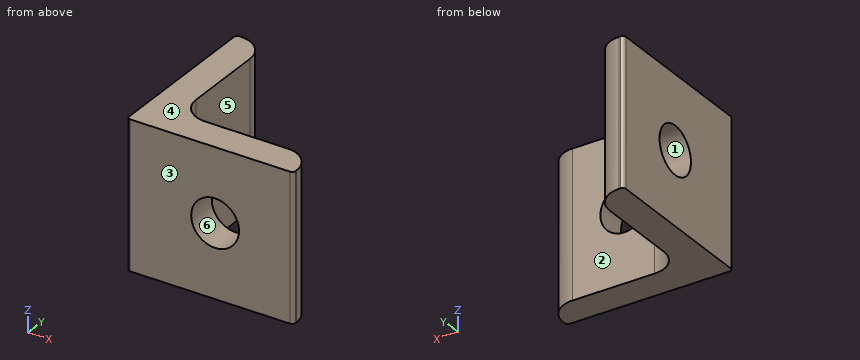
```python
from build123d import *

# Parameters (mm, degrees)
BOSS_EXTRUDE1_DEPTH = 22
SKETCH2_R           = 3.59
CUT_EXTRUDE1_DEPTH  = 42.641325627
SKETCH3_R           = 3.59
CUT_EXTRUDE2_DEPTH  = 42.641325627
FILLET1_R           = 4
FILLET2_R           = 0.5


with BuildPart() as part:
    # Sketch1 → Boss-Extrude1 (new body)
    with BuildSketch(Plane.XY):
        Polygon((0, 0), (25, 0), (25, 4.7), (4.7, 4.7), (4.7, 25), (0, 25), align=None)
    extrude(amount=BOSS_EXTRUDE1_DEPTH)

    # Sketch2 → Cut-Extrude1 (cut, through all)
    with BuildSketch(Plane.XZ):
        with Locations(Location((13.25, 11, 0), (0, 0, 270))):
            Circle(SKETCH2_R)
    extrude(amount=-CUT_EXTRUDE1_DEPTH, mode=Mode.SUBTRACT)

    # Sketch3 → Cut-Extrude2 (cut, through all)
    with BuildSketch(Plane.ZY):
        with Locations(Location((11, 13.25, 0), (0, 0, 270))):
            Circle(SKETCH3_R)
    extrude(amount=-CUT_EXTRUDE2_DEPTH, mode=Mode.SUBTRACT)

    # Fillet1
    fillet1_edges = [part.edges().sort_by_distance(p)[0] for p in [
        (4.7, 25, 11),
        (4.7, 4.7, 11),
        (25, 4.7, 11),
    ]]
    fillet(fillet1_edges, radius=FILLET1_R)

    # Fillet2
    fillet2_edges = [part.edges().sort_by_distance(p)[0] for p in [
        (0, 25, 11),
        (25, 0, 11),
        (0, 0, 11),
    ]]
    fillet(fillet2_edges, radius=FILLET2_R)


solid = part.part
```
Input: part model. Units: mm. Frame: model coordinates. Face numbers are marked on the shaded views. A direction names the side the tool comes from. Round coordinates to 2 decimals unless told otherwise and drop trailing zeros. Order: outer loops, then holes, each group sorted by start corner. A loop starts at its lowest first (then second) coordinate and runs counter-clockwise, first axis right, second up. Notation, with made-up numbers: (42.5, 25) - (78.5, 25) arc R27 ccw to (78.5, 55) - close; hole circle Ø5 at (-9.5, -13.75). An arc over 180 degrees is marked (long way). Answer in a Markdown table with one row per item.
Item 1: Pin query (flat end, axial travel): pin 1 (6 mm diameter, centred on x = 17, z = 11.5, fed in from +Y); pin 2 (3 mm diameter, centred on y = 2.5, z = 11.5, fed in from +X); pin 3 (8 mm diameter, centred on y = 19.5, z = 6, fed in from +X). Return the tip coordinate at first contact, or that it passes through.
Model answer:
| item | result |
|---|---|
| pin 1 | stops at y = 4.7 |
| pin 2 | stops at x = 24.99 |
| pin 3 | stops at x = 4.7 |
Item 2: Mould query, pull axis Y, two halves, no side actions, for the marked faces 1, 2, 3 and 4. Classes: released by +Y, released by -Y, zero draft, split by the parting line, or undercut.
Model answer:
| item | result |
|---|---|
| face 1 | undercut |
| face 2 | released by +Y |
| face 3 | released by -Y |
| face 4 | zero draft |
Item 3: Section query A-A (y = 13.25). Return the cut outline in (x, z), then the cut area to 3 significant figures.
Model answer:
| item | result |
|---|---|
| outline | (0, 0) - (4.7, 0) - (4.7, 7.41) - (0, 7.41) - close; (0, 14.59) - (4.7, 14.59) - (4.7, 22) - (0, 22) - close |
| area | 69.7 mm² |
Item 4: Line query: line 1 (Z direction, x = 3.5, y = 13.25); line 2 (Y direction, x = 15, z = 6.25). Output: solid intervals per line, ascending.
Model answer:
| item | result |
|---|---|
| line 1 | z = 0 to 7.41, 14.59 to 22 |
| line 2 | y = 0 to 4.7 |
Item 5: Section query B-B (z = 11). Return the cut outline in (x, y).
Model answer:
| item | result |
|---|---|
| outline | (0, 0.5) arc R0.5 ccw to (0.5, 0) - (9.66, 0) - (9.66, 4.7) - (8.7, 4.7) arc R4 cw to (4.7, 8.7) - (4.7, 9.66) - (0, 9.66) - close; (0, 16.84) - (4.7, 16.84) - (4.7, 21) arc R4 ccw to (0.7, 25) - (0.5, 25) arc R0.5 ccw to (0, 24.5) - close; (16.84, 0) - (24.5, 0) arc R0.5 ccw to (25, 0.5) - (25, 0.7) arc R4 ccw to (21, 4.7) - (16.84, 4.7) - close |
Item 6: Reachability of the marked faces 5 and 6 from +Z, -Z, +X, -X, +Y, -Y: full face, straight path, thin tool, end or side. Return the list, or none.
Model answer:
| item | result |
|---|---|
| face 5 | +Z, -Z, +X, +Y |
| face 6 | +Y, -Y |
Item 7: Section query D-D (z = 15.5). Return the cut outline in (x, y).
Model answer:
| item | result |
|---|---|
| outline | (0, 0.5) arc R0.5 ccw to (0.5, 0) - (24.5, 0) arc R0.5 ccw to (25, 0.5) - (25, 0.7) arc R4 ccw to (21, 4.7) - (8.7, 4.7) arc R4 cw to (4.7, 8.7) - (4.7, 21) arc R4 ccw to (0.7, 25) - (0.5, 25) arc R0.5 ccw to (0, 24.5) - close |
